Here's how the part is built. I have some questions about the finished solid (model axes, mm). A direction names the side the tool comes from. Give positions to 0.01 mm unless a question says otherwise; leave off trailing zeros. Write each loop counter-clockwise with the first axis right and the second up, starting at its lowest first coordinate (ties: lowest second). Pieces come first, ordered by that corner, then holes. Notation, with made-up numbers: (-19, -38) -> (18, -38) arc R19 ccw to (18, -14) -> close; hole circle Ø7 at (33, 10). An arc over 180 degrees is marked (long way). Put each result on its own line as item: value. Start each with the question number.
Autodesk Inventor part; units mm, degrees
ref_plane "YZ Plane" through (0, 0, 0) normal (1, 0, 0) x (0, 1, 0)
ref_plane "XZ Plane" through (0, 0, 0) normal (0, 1, 0) x (-1, 0, 0)
ref_plane "XY Plane" through (0, 0, 0) normal (0, 0, 1) x (1, 0, 0)
sketch "Sketch1" plane through (0, 0, 0) normal (1, 0, 0) x (0, 1, 0)
  line L0 (0, 0) -> (10, 0)
  line L1 (10, 0) -> (10, -10)
  line L2 (10, -10) -> (0, -10)
  line L3 (0, -10) -> (0, 0)
  dimension "d0" = 10
  dimension "d1" = 10
extrude "Extrusion1" add sketch "Sketch1" along normal blind 10
sketch "Sketch3" plane through (0, 0, 0) normal (-1, 0, 0) x (0, 0, 1)
  circle A0 centre (-5, 5) radius 1.5
  point P0 (0, 0)
extrude "Extrusion3" cut sketch "Sketch3" against normal blind 5
sketch "Sketch4" plane through (0, 0, 0) normal (0, 0, 1) x (1, 0, 0)
  line L0 (1.8731, 7.9408) -> (4.4271, 7.9408) construction
  line L1 (4.4271, 7.9408) -> (4.4271, 4.8928) construction
  line L2 (4.4271, 4.8928) -> (1.8731, 4.8928) construction
  line L3 (1.8731, 4.8928) -> (1.8731, 7.9408) construction
  spline S0 degree 2 poles (6.0379, 6.4263) (5.7961, 6.4263) (5.6751, 6.7102) knots 0 0 0 1 1 1
  spline S1 degree 2 poles (5.6751, 6.7102) (5.5699, 6.9521) (5.4805, 7.0047) knots 0 0 0 1 1 1
  spline S2 degree 2 poles (5.4805, 7.0047) (5.4017, 7.0468) (5.0861, 7.0468) knots 0 0 0 1 1 1
  spline S3 degree 2 poles (5.0861, 7.0468) (4.5392, 7.0468) (3.8714, 6.2107) knots 0 0 0 1 1 1
  spline S4 degree 2 poles (3.8714, 6.2107) (2.9669, 5.0853) (2.9669, 4.0809) knots 0 0 0 1 1 1
  spline S5 degree 2 poles (2.9669, 4.0809) (2.9669, 3.5919) (3.2824, 3.2448) knots 0 0 0 1 1 1
  spline S6 degree 2 poles (3.2824, 3.2448) (3.6032, 2.882) (4.0554, 2.882) knots 0 0 0 1 1 1
  spline S7 degree 2 poles (4.0554, 2.882) (4.4446, 2.882) (4.8337, 3.0818) knots 0 0 0 1 1 1
  spline S8 degree 2 poles (4.8337, 3.0818) (5.0546, 3.1975) (5.5068, 3.5288) knots 0 0 0 1 1 1
  spline S9 degree 2 poles (5.5068, 3.5288) (5.7224, 3.6865) (5.8329, 3.6865) knots 0 0 0 1 1 1
  spline S10 degree 2 poles (5.8329, 3.6865) (5.9906, 3.6865) (6.2115, 3.4394) (6.2115, 3.2921) knots 0 0 0 1 2 2 2
  spline S11 degree 2 poles (6.2115, 3.2921) (6.2115, 3.1186) (6.0695, 2.9924) knots 0 0 0 1 1 1
  spline S12 degree 2 poles (6.0695, 2.9924) (5.0704, 2.1089) (4.0554, 2.1089) knots 0 0 0 1 1 1
  spline S13 degree 2 poles (4.0554, 2.1089) (3.2719, 2.1089) (2.7355, 2.7084) knots 0 0 0 1 1 1
  spline S14 degree 2 poles (2.7355, 2.7084) (2.2149, 3.2869) (2.2149, 4.0809) knots 0 0 0 1 1 1
  spline S15 degree 2 poles (2.2149, 4.0809) (2.2149, 5.3588) (3.2877, 6.6997) knots 0 0 0 1 1 1
  spline S16 degree 2 poles (3.2877, 6.6997) (4.1817, 7.8198) (5.0861, 7.8198) knots 0 0 0 1 1 1
  spline S17 degree 2 poles (5.0861, 7.8198) (5.2702, 7.8198) (5.5647, 7.7883) (5.6804, 7.7462) knots 0 0 0 1 2 2 2
  spline S18 degree 2 poles (5.6804, 7.7462) (5.8118, 7.9408) (6.0222, 7.9408) knots 0 0 0 1 1 1
  spline S19 degree 2 poles (6.0222, 7.9408) (6.2851, 7.9408) (6.3535, 7.5989) knots 0 0 0 1 1 1
  spline S20 degree 2 poles (6.3535, 7.5989) (6.4113, 7.2887) (6.4113, 6.847) knots 0 0 0 1 1 1
  spline S21 degree 2 poles (6.4113, 6.847) (6.4113, 6.6892) (6.3272, 6.5735) knots 0 0 0 1 1 1
  spline S22 degree 2 poles (6.3272, 6.5735) (6.2273, 6.4263) (6.0379, 6.4263) knots 0 0 0 1 1 1
  point P0 (0, 0)
extrude "Extrusion4" cut sketch "Sketch4" against normal blind 2
properties part number "Cytosine"
1) I want a section at B-B, the plane x = 1.25. Write out the boundary of the cut face in (y, z), and give its area (3 significant figures).
2) I need wall thicknesses on probe 1 along Y at (x, z) = (2.7, -5); probe 2 along Z at (x, y) = (3.5, 2.5); probe 3 along Z at (x, y) = (1.25, 4.5). Which ranges of each line are inside material? Lowest first, please.
3) Which directions (+Z, -Z, +X, -X, +Y, -Y) give clear straight access to the entire face, cutting with the end or side of a thin tool? Please do faces 5 (the flat face through (0, 3.8, -3.8)), 6 (the flat face through (3.1, 5.3, -2)).
4) Thinking about a two-plate mould opening in Z: for faces 1 (the cylindrical face through (2.5, 4.1, -6.2)), 2 (the flat face through (10, 5, -5)), 3 (the flat face through (5, 5, 0)), 4 (the flat face through (5, 5, -5)), which applies, released by +Z, released by -Z, zero draft, split by the parting line, or undercut?
5) I want a section at A-A, the plane z = -5. Write out the boundary of the cut face in (x, y), and give its area (3 significant figures).
Established:
1. outline: (0, -10) -> (10, -10) -> (10, 0) -> (0, 0) -> close; hole circle Ø3 at (5, -5)
1. area: 92.9 mm2
2. probe 1: y = 0 to 3.5, 6.5 to 10
2. probe 2: z = -10 to -2
2. probe 3: z = -10 to -6.41, -3.59 to 0
3. face 5: +Z, -Z, -X, +Y, -Y
3. face 6: +Z
4. face 1: undercut
4. face 2: zero draft
4. face 3: released by +Z
4. face 4: undercut
5. outline: (0, 0) -> (10, 0) -> (10, 10) -> (0, 10) -> (0, 6.5) -> (5, 6.5) -> (5, 3.5) -> (0, 3.5) -> close
5. area: 85.0 mm2
